```python
from build123d import *

# Parameters (mm, degrees)
SKETCH1_W           = 30
SKETCH1_H           = 40
SKETCH1_R           = 4.25
BOSS_EXTRUDE1_DEPTH = 1.5
SKETCH2_W           = 40
SKETCH2_H           = 30.5
BOSS_EXTRUDE2_DEPTH = 1.5
SKETCH3_W           = 11.5
SKETCH3_H           = 40
SKETCH3_R           = 1.75
BOSS_EXTRUDE3_DEPTH = 1.5
FILLET1_R           = 1
FILLET2_R           = 3


with BuildPart() as part:
    # Sketch1 → Boss-Extrude1 (new body)
    with BuildSketch(Plane(origin=(0, 0, 0), x_dir=(1, 0, 0), z_dir=(0, 1, 0))):
        Rectangle(SKETCH1_W, SKETCH1_H)
        Circle(SKETCH1_R, mode=Mode.SUBTRACT)
    extrude(amount=BOSS_EXTRUDE1_DEPTH)

    # Sketch2 → Boss-Extrude2 (add)
    with BuildSketch(Plane.ZY.offset(15)):
        with Locations((0, 15.25)):
            Rectangle(SKETCH2_W, SKETCH2_H)
    boss_extrude2 = extrude(amount=-BOSS_EXTRUDE2_DEPTH)

    # Sketch3 → Boss-Extrude3 (add)
    with BuildSketch(Plane(origin=(0, 30.5, 0), x_dir=(1, 0, 0), z_dir=(0, 1, 0))):
        with Locations((-19.25, 0)):
            Rectangle(SKETCH3_W, SKETCH3_H)
        with Locations((-20, 15)):
            Circle(SKETCH3_R, mode=Mode.SUBTRACT)
        with Locations((-20, -15)):
            Circle(SKETCH3_R, mode=Mode.SUBTRACT)
    boss_extrude3 = extrude(amount=-BOSS_EXTRUDE3_DEPTH)

    # Mirror1: Boss-Extrude2, Boss-Extrude3 across plane
    add(boss_extrude2.mirror(Plane(origin=(0, 0, 0), x_dir=(0, 0, 1), z_dir=(1, 0, 0))))
    add(boss_extrude3.mirror(Plane(origin=(0, 0, 0), x_dir=(0, 0, 1), z_dir=(1, 0, 0))))

    # Fillet1
    fillet1_edges = [part.edges().sort_by_distance(p)[0] for p in [
        (-13.5, 1.5, 0),
        (-15, 29, 0),
        (15, 0, 0),
        (-15, 0, 0),
        (13.5, 1.5, 0),
        (15, 29, 0),
    ]]
    fillet(fillet1_edges, radius=FILLET1_R)

    # Fillet2
    fillet2_edges = [part.edges().sort_by_distance(p)[0] for p in [
        (-25, 29.75, -20),
        (-25, 29.75, 20),
        (25, 29.75, 20),
        (25, 29.75, -20),
    ]]
    fillet(fillet2_edges, radius=FILLET2_R)


solid = part.part
```
Could you check a few things on this model? Use its own coordinates, in mm. A direction names the side the tool comes from. Give positions to 0.01 mm unless a question says otherwise; leave off trailing zeros. Order: outer loops, then holes, each group sorted by start corner. A loop starts at its lowest first (then second) coordinate and runs counter-clockwise, first axis right, second up.
Q1. Suppose I cut it at A-A, the plane z = 0. Write out the boundary of the cut face in (x, y).
Q2. For faces 1 (the flat face through (21, 29, 0)), 2 (the cylindrical face through (21.29, 29.76, 13.82)), 3 (the flat face through (-21, 29, 0)), 4 (the flat face through (-13.5, 17, 0)), which set-ups out of +Z, -Z, +X, -X, +Y, -Y let a thin tool reach every point of the face, with its end or its side?
Q3. Suppose I cut it at B-B, the plane y = 4. Write out the boundary of the cut face in (x, z), and give its area (3 significant figures).
Q4. Suppose I cut it at C-C, the plane x = 20. Write out the boundary of the cut face in (y, z), and give its area (3 significant figures).
Q5. I'm going to push flat-ended pins straight in: P1, Ø4, axis at x = 20, z = -15, coming from the +Y side; P2, Ø2.5, axis at x = 19.5, z = -9, coming from the -Y side; P3, Ø1.5, axis at x = 1, y = 3.5, coming from the -Z side; P4, Ø4, axis at y = 9.5, z = -7.5, coming from the -X side. Where does each tip first touch, or does it pass through?
Q6. If I drill on line 1 along Z through (x, y) = (-20, 29.7); line 2 along X through (y, z) = (29.4, -15); line 3 along X through (y, z) = (6.5, 13.5), over which ranges is the centre line in solid material (lowest first)?
Q7. Suppose I cut it at D-D, the plane z = -15. Write out the boundary of the cut face in (x, y).
Solution:
1. outline: (-25, 29) - (-16, 29) arc R1 cw to (-15, 28) - (-15, 1) arc R1 ccw to (-14, 0) - (-4.25, 0) - (-4.25, 1.5) - (-12.5, 1.5) arc R1 cw to (-13.5, 2.5) - (-13.5, 30.5) - (-25, 30.5) - close; (4.25, 0) - (14, 0) arc R1 ccw to (15, 1) - (15, 28) arc R1 cw to (16, 29) - (25, 29) - (25, 30.5) - (13.5, 30.5) - (13.5, 2.5) arc R1 cw to (12.5, 1.5) - (4.25, 1.5) - close
2. face 1: +Z, -Z, +X, -Y
2. face 2: +Y, -Y
2. face 3: +Z, -Z, -X, -Y
2. face 4: +Z, -Z, +Y
3. outline: (-15, -20) - (-13.5, -20) - (-13.5, 20) - (-15, 20) - close; (13.5, -20) - (15, -20) - (15, 20) - (13.5, 20) - close
3. area: 120 mm2
4. outline: (29, -20) - (30.5, -20) - (30.5, -16.75) - (29, -16.75) - close; (29, -13.25) - (30.5, -13.25) - (30.5, 13.25) - (29, 13.25) - close; (29, 16.75) - (30.5, 16.75) - (30.5, 20) - (29, 20) - close
4. area: 49.5 mm2
5. P1: stops at y = 30.5
5. P2: stops at y = 29
5. P3: passes through
5. P4: stops at x = -15
6. line 1: z = -20 to -16.75, -13.25 to 13.25, 16.75 to 20
6. line 2: x = -25 to -21.75, -18.25 to -13.5, 13.5 to 18.25, 21.75 to 25
6. line 3: x = -15 to -13.5, 13.5 to 15
7. outline: (-25, 29) - (-21.75, 29) - (-21.75, 30.5) - (-25, 30.5) - close; (-18.25, 29) - (-16, 29) arc R1 cw to (-15, 28) - (-15, 1) arc R1 ccw to (-14, 0) - (14, 0) arc R1 ccw to (15, 1) - (15, 28) arc R1 cw to (16, 29) - (18.25, 29) - (18.25, 30.5) - (13.5, 30.5) - (13.5, 2.5) arc R1 cw to (12.5, 1.5) - (-12.5, 1.5) arc R1 cw to (-13.5, 2.5) - (-13.5, 30.5) - (-18.25, 30.5) - close; (21.75, 29) - (25, 29) - (25, 30.5) - (21.75, 30.5) - close
